from build123d import *

# Parameters (mm, degrees)
EXTRUDE_1_DEPTH     = 6
CUT_EXTRUDE_5_DEPTH = 45.878603962
SKETCH_4_R          = 7.75
CUT_EXTRUDE_6_DEPTH = 35.872445467
FILLET_1_R          = 5
SKETCH_5_R          = 8.5
CUT_EXTRUDE_7_DEPTH = 1


with BuildPart() as part:
    # 草图1 → 凸台-拉伸1 (new body)
    with BuildSketch(Plane.XY):
        Polygon((-10.499999762, 10.5), (10.500000238, 10.5), (10.500000238, -10.500000475), (10.500000238, -32.718504007), (-10.499999762, -32.718504007), (-10.499999762, -10.499999525), align=None)
    extrude(amount=EXTRUDE_1_DEPTH)

    # 草图8 → 切除-拉伸5 (cut, through all)
    with BuildSketch(Plane(origin=(0, 10.5, 0), x_dir=(1, 0, 0), z_dir=(0, 1, 0))):
        with BuildLine():
            Line((-19.020487649, 0.47662404), (13.656545029, 0.844180338))
            add(Edge.make_bspline(
                [(-19.020487649, 0.47662404), (-14.907938577, -0.444262453), (-8.455698153, -1.333893864), (2.536876626, -1.118098726), (9.340479573, -0.673611335), (13.656545029, 0.844180338)],
                knots=[0, 0, 0, 0, 0.38369485, 0.588358138, 1, 1, 1, 1], degree=3))
        make_face()
    extrude(amount=-CUT_EXTRUDE_5_DEPTH, mode=Mode.SUBTRACT)

    # 草图4 → 切除-拉伸6 (cut, through all)
    with BuildSketch(Plane.XY.offset(6)):
        Circle(SKETCH_4_R)
    extrude(amount=-CUT_EXTRUDE_6_DEPTH, mode=Mode.SUBTRACT)

    # 圆角1
    fillet_1_edges = [part.edges().sort_by_distance(p)[0] for p in [
        (-10.499999762, -32.718504007, 3.451578548),
        (10.500000238, -32.718504007, 3.027756169),
        (10.500000238, 10.5, 3.027756169),
        (-10.499999762, 10.5, 3.451578548),
    ]]
    fillet(fillet_1_edges, radius=FILLET_1_R)

    # 草图5 → 切除-拉伸7 (cut)
    with BuildSketch(Plane.XY.offset(6)):
        Circle(SKETCH_5_R)
    extrude(amount=-CUT_EXTRUDE_7_DEPTH, mode=Mode.SUBTRACT)


solid = part.part
For this review, take the finished solid that the model builds, in its own axes (mm). A direction names the side the tool comes from. Give positions to 0.01 mm unless a question says otherwise; leave off trailing zeros. Order: outer loops, then holes, each group sorted by start corner. A loop starts at its lowest first (then second) coordinate and runs counter-clockwise, first axis right, second up. Notation, with made-up numbers: (79, 74) - (96, 74) arc R17 cw to (96, 100) - close; hole circle Ø6 at (44, 12.25). An arc over 180 degrees is marked (long way). Answer as a JSON object with one key per item and string values. Group by question number.
Item 1: Machinability: for faces 4 (the flat face through (8, 2, 5)), 5 (the flat face through (0, -32.719, 3)), which of the approach directions +Z, -Z, +X, -X, +Y, -Y give a long, thin tool a straight path to every point of the face, cutting with its end or side? Answer none if there is none.
Item 2: Clearance check with flat-ended pins moving along their axes: pin 1 Ø4 at (x, y) = (1.5, -25) entering from -Z; pin 2 Ø3 at (x, y) = (6, -3.5) entering from +Z. State where each tip first meets the part, or that it passes through.
Item 3: Take a section at A-A on z = 2. Give the boundary of the cut face in (x, y), and give its area (3 significant figures).
Item 4: Draft analysis for pull direction X (two halves, no side actions). For faces 1 (the cylindrical face through (4.57, 7.167, 5.507)), 2 (the cylindrical face through (-9, 9.07, 3.49)), 3 (the flat face through (10.5, -11, 3)), state which applies: pulls with the +X half, pulls with the -X half, needs draft (parallel to the pull), parting line crosses it, or undercut.
Item 5: Wall thickness on line 1 along Y through (x, z) = (0, 5.5); line 2 along Y through (x, z) = (0, 1.5); line 3 along X through (y, z) = (0, 2.9): over which ranges is each line inside the solid? List them lowest first.
Reported:
{
 "1": {"face 4": "+Z", "face 5": "+Z, -Z, +X, -X, -Y"},
 "2": {"pin 1": "z = 0.98", "pin 2": "z = 5"},
 "3": {"outline": "(-10.5, -27.72) arc R5 ccw to (-5.5, -32.72) - (5.5, -32.72) arc R5 ccw to (10.5, -27.72) - (10.5, 5.5) arc R5 ccw to (5.5, 10.5) - (-5.5, 10.5) arc R5 ccw to (-10.5, 5.5) - close; hole circle Ø15.5 at (0, 0)", "area": "697 mm^2"},
 "4": {"face 1": "undercut", "face 2": "pulls with the -X half", "face 3": "pulls with the +X half"},
 "5": {"line 1": "-32.72 to -8.5, 8.5 to 10.5", "line 2": "-32.72 to -7.75, 7.75 to 10.5", "line 3": "-10.5 to -7.75, 7.75 to 10.5"}
}
